from build123d import *

# Parameters (mm, degrees)
SKETCH_1_W                  = 260
SKETCH_1_H                  = 220
EXTRUDE_1_DEPTH             = 12
SKETCH_2_W                  = 2
SKETCH_2_H                  = 94
CUT_EXTRUDE_1_DEPTH         = 283.56680626
HOLE_WIZARD_1_D             = 5.5
HOLE_WIZARD_1_CBORE_D       = 10
HOLE_WIZARD_1_CBORE_DEPTH   = 5
HOLE_WIZARD_2_D             = 6.6
HOLE_WIZARD_2_CBORE_D       = 11
HOLE_WIZARD_2_CBORE_DEPTH   = 6.8
SKETCH_7_W                  = 37
SKETCH_7_H                  = 86
CUT_EXTRUDE_2_DEPTH         = 171.716138663
HOLE_WIZARD_M6_1_AT_2_COUNT = 2
HOLE_WIZARD_M6_1_AT_2_PITCH = 40
CUT_EXTRUDE_3_DEPTH         = 171.716138663
HOLE_WIZARD_M6_2_D          = 5


with BuildPart() as part:
    # 草图1 → 凸台-拉伸1 (new body)
    with BuildSketch(Plane.XY):
        Rectangle(SKETCH_1_W, SKETCH_1_H)
    extrude(amount=EXTRUDE_1_DEPTH)

    # 草图2 → 切除-拉伸1 (cut, through all)
    with BuildSketch(Plane(origin=(130, 0, 0), x_dir=(0, 0, -1), z_dir=(1, 0, 0))):
        with Locations((-1, -63)):
            Rectangle(SKETCH_2_W, SKETCH_2_H)
    extrude(amount=-CUT_EXTRUDE_1_DEPTH, mode=Mode.SUBTRACT)

    # 打孔尺寸根据内六角圆柱头螺钉的类型1 (through all)
    with Locations(Plane.XY.offset(12)):
        with Locations((-58, -22), (-22, -22), (-22, -54), (-58, -54), (58, -54), (22, -54), (22, -22), (58, -22), (58, -104), (22, -104), (22, -72), (58, -72), (-58, -72), (-22, -72), (-22, -104), (-58, -104)):
            CounterBoreHole(HOLE_WIZARD_1_D / 2, HOLE_WIZARD_1_CBORE_D / 2, HOLE_WIZARD_1_CBORE_DEPTH)

    # 打孔尺寸根据内六角圆柱头螺钉的类型2 (through all)
    with Locations(Plane.XY.offset(12)):
        with Locations((-124, 18), (0, 18), (124, 18)):
            CounterBoreHole(HOLE_WIZARD_2_D / 2, HOLE_WIZARD_2_CBORE_D / 2, HOLE_WIZARD_2_CBORE_DEPTH)

    # 草图7 → 切除-拉伸2 (cut, through all)
    with BuildSketch(Plane.XY.offset(12)):
        with Locations((111.5, 67)):
            Rectangle(SKETCH_7_W, SKETCH_7_H)
        with Locations((-111.5, 67)):
            Rectangle(SKETCH_7_W, SKETCH_7_H)
    extrude(amount=-CUT_EXTRUDE_2_DEPTH, mode=Mode.SUBTRACT)

    # 草图8 → M6 螺纹孔1 (revolve, cut)
    with BuildSketch(Plane(origin=(-93, 87, 6), x_dir=(0, 0, 1), z_dir=(0, 1, 0))):
        Polygon((0, 0), (0, 16.502151548), (2.5, 15), (2.5, 0), align=None)
    hole_wizard_m6_1 = revolve(axis=Axis((-99.35, 87, 6), (1, 0, 0)), mode=Mode.SUBTRACT)

    # M6 螺纹孔1 at 2: M6 螺纹孔1 ×2
    with Locations(*[(0, -i * HOLE_WIZARD_M6_1_AT_2_PITCH, 0) for i in range(1, HOLE_WIZARD_M6_1_AT_2_COUNT)]):
        add(hole_wizard_m6_1, mode=Mode.SUBTRACT)

    # 镜向1: M6 螺纹孔1 across plane
    add(hole_wizard_m6_1.mirror(Plane(origin=(0, 0, 0), x_dir=(0, 0, 1), z_dir=(1, 0, 0))), mode=Mode.SUBTRACT)

    # 镜向1 copy 1 sketch → 镜向1 copy 1 (revolve, cut)
    with BuildSketch(Plane(origin=(93, 47, 6), x_dir=(0, 0, 1), z_dir=(0, 1, 0))):
        Polygon((0, 0), (0, -16.502151548), (2.5, -15), (2.5, 0), align=None)
    revolve(axis=Axis((99.35, 47, 6), (1, 0, 0)), mode=Mode.SUBTRACT)

    # 草图10 → 切除-拉伸3 (cut, through all)
    with BuildSketch(Plane.XY.offset(12)):
        with BuildLine():
            Line((-88, -101), (-82, -101))
            ThreePointArc((-82, -101), (-78.464466094, -99.535533906), (-77, -96))
            Line((-77, -96), (-77, -30))
            ThreePointArc((-77, -30), (-78.464466094, -26.464466094), (-82, -25))
            Line((-82, -25), (-88, -25))
            ThreePointArc((-88, -25), (-91.535533906, -26.464466094), (-93, -30))
            Line((-93, -30), (-93, -96))
            ThreePointArc((-93, -96), (-91.535533906, -99.535533906), (-88, -101))
        make_face()
        with BuildLine():
            Line((-72, 64), (72, 64))
            ThreePointArc((72, 64), (75.535533906, 62.535533906), (77, 59))
            Line((77, 59), (77, 29))
            ThreePointArc((77, 29), (75.535533906, 25.464466094), (72, 24))
            Line((72, 24), (-72, 24))
            ThreePointArc((-72, 24), (-75.535533906, 25.464466094), (-77, 29))
            Line((-77, 29), (-77, 59))
            ThreePointArc((-77, 59), (-75.535533906, 62.535533906), (-72, 64))
        make_face()
        with BuildLine():
            Line((77, -96), (77, -30))
            ThreePointArc((77, -30), (78.464466094, -26.464466094), (82, -25))
            Line((82, -25), (88, -25))
            ThreePointArc((88, -25), (91.535533906, -26.464466094), (93, -30))
            Line((93, -30), (93, -96))
            ThreePointArc((93, -96), (91.535533906, -99.535533906), (88, -101))
            Line((88, -101), (82, -101))
            ThreePointArc((82, -101), (78.464466094, -99.535533906), (77, -96))
        make_face()
    extrude(amount=-CUT_EXTRUDE_3_DEPTH, mode=Mode.SUBTRACT)

    # M6 螺纹孔2 (through all)
    with Locations(Plane.XY.offset(12)):
        with Locations((-99, -10), (-99, -100), (99, -100), (99, -10)):
            Hole(HOLE_WIZARD_M6_2_D / 2)

    # 草图13 → M4 螺纹孔1 (revolve, cut)
    with BuildSketch(Plane(origin=(-130, -90, 6), x_dir=(0, 0, 1), z_dir=(0, 1, 0))):
        Polygon((0, 0), (0, 11.091420021), (1.65, 10.1), (1.65, 0), align=None)
    hole_wizard_m4_1 = revolve(axis=Axis((-136.35, -90, 6), (1, 0, 0)), mode=Mode.SUBTRACT)

    # 镜向2: M4 螺纹孔1 across plane
    add(hole_wizard_m4_1.mirror(Plane(origin=(0, 0, 0), x_dir=(0, 0, 1), z_dir=(1, 0, 0))), mode=Mode.SUBTRACT)


solid = part.part
Can you work these out from the model? Positions are in its coordinate system, mm. A direction names the side the tool comes from. Round coordinates to 2 decimals unless told otherwise and drop trailing zeros. Loops run counter-clockwise (first coordinate to the right, second up) from the corner with the lowest first, then second, coordinate; pieces in that order, holes last. Notation, with made-up numbers: (74.5, 33.5) - (98.5, 33.5) arc R24 ccw to (98.5, 70.5) - close; hole circle Ø9 at (-37, 59.25). An arc over 180 degrees is marked (long way). Answer in a Markdown table with one row per item. Add a question column.
Q1. I want a section at A-A on x = 124. List the corners of the cut face in (y, z) for me.
Q2. For pin 1 Ø6.5 at (x, y) = (58, -22) entering from +Z; pin 2 Ø2 at (x, y) = (-16.5, -71.5) entering from -Z; pin 3 Ø1 at (y, z) = (72.5, 6.5) entering from -X, each with a flat end and sliding along its axis, tell me the tip position at first contact or that it passes through.
Q3. I need wall thicknesses on L1, parallel to Y at x = 22, z = 5.6; L2, parallel to X at y = -35, z = 2.75; L3, parallel to Y at x = 58, z = 10.5. Which ranges of each line are inside material? Lowest first, please.
Q4. I want a section at B-B on y = -43. List the corners of the cut face in (x, z) for me, and give its area (3 significant figures).
Q5. I want a section at C-C on x = 50. List the corners of the cut face in (y, z) for me, and give its area (3 significant figures).
Q6. Which directions (+Z, -Z, +X, -X, +Y, -Y) give clear straight access to the entire face, cutting with the end or side of a thin tool? Please do faces 1 (the flat face through (-93, 66, 6)), 2 (the flat face through (124, 14, 5.2)), 3 (the cylindrical face through (24.027, -70.141, 4.465)).
A:
| question | item | result |
|---|---|---|
| 1 | outline | (-110, 2) - (-16, 2) - (-16, 0) - (14.7, 0) - (14.7, 5.2) - (12.5, 5.2) - (12.5, 12) - (-110, 12) - close; (21.3, 0) - (24, 0) - (24, 12) - (23.5, 12) - (23.5, 5.2) - (21.3, 5.2) - close; hole circle Ø3.3 at (-90, 6) |
| 2 | pin 1 | z = 7 |
| 2 | pin 2 | z = 2 |
| 2 | pin 3 | x = -93 |
| 3 | L1 | -110 to -106.75, -101.25 to -74.75, -69.25 to -56.75, -51.25 to -24.75, -19.25 to 24, 64 to 110 |
| 3 | L2 | -130 to -93, -77 to 77, 93 to 130 |
| 3 | L3 | -110 to -109, -99 to -77, -67 to -59, -49 to -27, -17 to 24, 64 to 110 |
| 4 | outline | (-130, 2) - (-93, 2) - (-93, 12) - (-130, 12) - close; (-77, 2) - (77, 2) - (77, 12) - (-77, 12) - close; (93, 2) - (130, 2) - (130, 12) - (93, 12) - close |
| 4 | area | 2,280 mm^2 |
| 5 | outline | (-110, 2) - (-16, 2) - (-16, 0) - (24, 0) - (24, 12) - (-110, 12) - close; (64, 0) - (110, 0) - (110, 12) - (64, 12) - close |
| 5 | area | 1,970 mm^2 |
| 6 | face 1 | +Z, -Z, -X, +Y |
| 6 | face 2 | +Z |
| 6 | face 3 | +Z, -Z |
